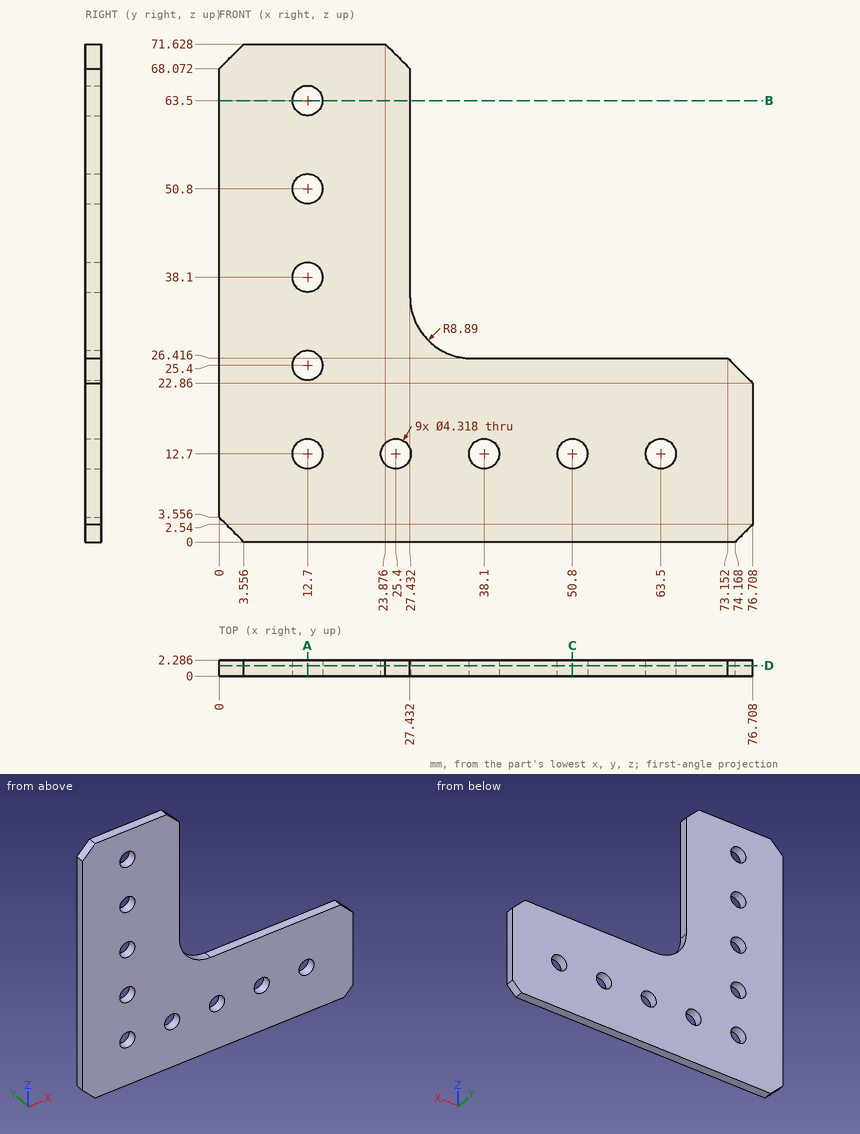
Geometry check sheet. Reference: drawing and pictorial views, mm from the part's lowest x, y, z. Round coordinates to 2 decimals unless told otherwise and drop trailing zeros. Loops run counter-clockwise (first coordinate to the right, second up) from the corner with the lowest first, then second, coordinate; pieces in that order, holes last.
1. Gauge pin test, flat ends, axial feed: pin 1 Ø4 at (x, z) = (38.1, 12.7) entering from +Y (3 decimals); pin 2 Ø0.7 at (x, y) = (50, 0.5) entering from +Z. Record the tip position at first contact, or that the pin passes through.
2. Sectioned sample at A-A on x = 12.7. Record the boundary of the cut face in (y, z), and give its area (3 significant figures).
3. Sectioned sample at C-C on x = 50.8. Record the boundary of the cut face in (y, z).
4. Sectioned sample at B-B on z = 63.5. Record the boundary of the cut face in (x, y).
5. Scan lines: probe 1 along Z at (x, y) = (12.7, 1.7); probe 2 along Z at (x, y) = (50.8, 0.75); probe 3 along Z at (x, y) = (56, 0.9). Record each from-to range of solid material in increasing order.
6. Sectioned sample at D-D on y = 1.5. Give the number of separate pieces and of enclosed holes in the cut face, and give its area (3 significant figures).
Recorded:
1. pin 1: passes through
1. pin 2: stops at z = 26.42
2. outline: (0, 0) - (2.29, 0) - (2.29, 10.54) - (0, 10.54) - close; (0, 14.86) - (2.29, 14.86) - (2.29, 23.24) - (0, 23.24) - close; (0, 27.56) - (2.29, 27.56) - (2.29, 35.94) - (0, 35.94) - close; (0, 40.26) - (2.29, 40.26) - (2.29, 48.64) - (0, 48.64) - close; (0, 52.96) - (2.29, 52.96) - (2.29, 61.34) - (0, 61.34) - close; (0, 65.66) - (2.29, 65.66) - (2.29, 71.63) - (0, 71.63) - close
2. area: 114 mm2
3. outline: (0, 0) - (2.29, 0) - (2.29, 10.54) - (0, 10.54) - close; (0, 14.86) - (2.29, 14.86) - (2.29, 26.42) - (0, 26.42) - close
4. outline: (0, 0) - (10.54, 0) - (10.54, 2.29) - (0, 2.29) - close; (14.86, 0) - (27.43, 0) - (27.43, 2.29) - (14.86, 2.29) - close
5. probe 1: z = 0 to 10.54, 14.86 to 23.24, 27.56 to 35.94, 40.26 to 48.64, 52.96 to 61.34, 65.66 to 71.63
5. probe 2: z = 0 to 10.54, 14.86 to 26.42
5. probe 3: z = 0 to 26.42
6. separate pieces: 1
6. enclosed holes: 9
6. area: 3,120 mm2
